from build123d import *

# Parameters (mm, degrees)
EXTRUDE_1_DEPTH     = 300
SKETCH_2_R          = 6
CUT_EXTRUDE_1_DEPTH = 300
SKETCH_3_R          = 2
CUT_EXTRUDE_2_DEPTH = 300


with BuildPart() as part:
    # 草图1 → 凸台-拉伸1 (new body)
    with BuildSketch(Plane.XY):
        Polygon((-15, -15), (15, -15), (15, 15), (12, 15), (12, -12), (-15, -12), align=None)
    extrude(amount=EXTRUDE_1_DEPTH)

    # 草图2 → 切除-拉伸1 (cut)
    with BuildSketch(Plane.ZY.offset(-12)):
        with Locations((20, 3)):
            Circle(SKETCH_2_R)
        with Locations((85, 3)):
            Circle(SKETCH_2_R)
        with Locations((150, 3)):
            Circle(SKETCH_2_R)
        with Locations((215, 3)):
            Circle(SKETCH_2_R)
        with Locations((280, 3)):
            Circle(SKETCH_2_R)
    extrude(amount=-CUT_EXTRUDE_1_DEPTH, mode=Mode.SUBTRACT)

    # 草图3 → 切除-拉伸2 (cut)
    with BuildSketch(Plane.XZ.offset(15)):
        with Locations(Location((-8, 295, 0), (0, 0, 270))):
            Circle(SKETCH_3_R)
        with Locations(Location((-8, 279, 0), (0, 0, 270))):
            Circle(SKETCH_3_R)
        with Locations(Location((8, 279, 0), (0, 0, 270))):
            Circle(SKETCH_3_R)
        with Locations(Location((8, 295, 0), (0, 0, 270))):
            Circle(SKETCH_3_R)
        with Locations(Location((-8, 21, 0), (0, 0, 270))):
            Circle(SKETCH_3_R)
        with Locations(Location((-8, 5, 0), (0, 0, 270))):
            Circle(SKETCH_3_R)
        with Locations(Location((8, 5, 0), (0, 0, 270))):
            Circle(SKETCH_3_R)
        with Locations(Location((8, 21, 0), (0, 0, 270))):
            Circle(SKETCH_3_R)
    extrude(amount=-CUT_EXTRUDE_2_DEPTH, mode=Mode.SUBTRACT)


solid = part.part
Design review of the part built by this model. Coordinates are the model's own, in mm. A direction names the side the tool comes from. Round coordinates to 2 decimals unless told otherwise and drop trailing zeros. Write each loop counter-clockwise with the first axis right and the second up, starting at its lowest first coordinate (ties: lowest second). Pieces come first, ordered by that corner, then holes.
Item 1: Consider section C-C on z = 239. Give the boundary of the cut face in (x, y), and give its area (3 significant figures).
Item 2: For pin 1 Ø11 at (y, z) = (3, 150) entering from -X; pin 2 Ø12 at (y, z) = (0.5, 223.5) entering from -X; pin 3 Ø13.5 at (x, z) = (4.5, 167.5) entering from +Y, all flat-tipped, find the tip position at first contact; note any pin that passes through.
Item 3: Draft analysis for pull direction Z (two halves, no side actions). For faces 3 (the flat face through (6.6, -12.2, 300)), 4 (the cylindrical face through (13.48, -0.65, 210.24)), 5 (the flat face through (15, -4, 148)), state which applies: released by +Z, released by -Z, zero draft, split by the parting line, or undercut.
Item 4: Wall thickness on L1, parallel to X at y = -14.2, z = 279; L2, parallel to X at y = 4, z = 69; L3, parallel to Y at x = 10, z = 225.5: over which ranges is each line inside the solid? List them lowest first.
Item 5: Consider section B-B on y = 3. Give the boundary of the cut face in (x, z).
Item 6: Consider section A-A on z = 150. Give the boundary of the cut face in (x, y), and give its area (3 significant figures).
Item 7: Consider section D-D on x = 2. Give the boundary of the cut face in (y, z), and give its area (3 significant figures).
Item 8: For faces 1 (the cylindrical face through (13.48, -0.65, 145.24)), 2 (the flat face through (-1, -12, 148)), list the 3-axis set-ups (+Z, -Z, +X, -X, +Y, -Y) from which the entire face can be reached by the end or side of a thin tool; tool diameter is ignored.
Check values:
1. outline: (-15, -15) - (15, -15) - (15, 15) - (12, 15) - (12, -12) - (-15, -12) - close
1. area: 171 mm2
2. pin 1: passes through
2. pin 2: stops at x = 12
2. pin 3: stops at y = -12
3. face 3: released by +Z
3. face 4: undercut
3. face 5: zero draft
4. L1: x = -15 to -10, -6 to 6, 10 to 15
4. L2: x = 12 to 15
4. L3: y = -15 to -12
5. outline: (12, 0) - (15, 0) - (15, 14) - (12, 14) - close; (12, 26) - (15, 26) - (15, 79) - (12, 79) - close; (12, 91) - (15, 91) - (15, 144) - (12, 144) - close; (12, 156) - (15, 156) - (15, 209) - (12, 209) - close; (12, 221) - (15, 221) - (15, 274) - (12, 274) - close; (12, 286) - (15, 286) - (15, 300) - (12, 300) - close
6. outline: (-15, -15) - (15, -15) - (15, -3) - (12, -3) - (12, -12) - (-15, -12) - close; (12, 9) - (15, 9) - (15, 15) - (12, 15) - close
6. area: 135 mm2
7. outline: (-15, 0) - (-12, 0) - (-12, 300) - (-15, 300) - close
7. area: 900 mm2
8. face 1: +X, -X
8. face 2: +Z, -Z, -X, +Y
